from build123d import *

# Parameters (mm, degrees)
SKETCH_1_W      = 215
SKETCH_1_H      = 43.5
EXTRUDE_1_DEPTH = 26
SKETCH_2_W      = 12
SKETCH_2_H      = 20
SKETCH_2_R      = 3.5
EXTRUDE_2_DEPTH = 5
SKETCH_3_R      = 4.2
EXTRUDE_3_DEPTH = 25


with BuildPart() as part:
    # ｽｹｯﾁ1 → ﾎﾞｽ - 押し出し1 (new body)
    with BuildSketch(Plane(origin=(0, 0, 0), x_dir=(1, 0, 0), z_dir=(0, 1, 0))):
        Rectangle(SKETCH_1_W, SKETCH_1_H)
    extrude(amount=EXTRUDE_1_DEPTH)

    # ｽｹｯﾁ2 → ﾎﾞｽ - 押し出し2 (add)
    # profile 1 of 2: a face of its own
    with BuildSketch(Plane.XZ):
        with Locations((-113.5, 0)):
            Rectangle(SKETCH_2_W, SKETCH_2_H)
        with Locations(Location((-113.5, 0, 0), (0, 0, 270))):
            Circle(SKETCH_2_R, mode=Mode.SUBTRACT)
    # profile 2 of 2: a face of its own
    with BuildSketch(Plane.XZ):
        with Locations((113.5, 0)):
            Rectangle(SKETCH_2_W, SKETCH_2_H)
        with Locations(Location((113.5, 0, 0), (0, 0, 90))):
            Circle(SKETCH_2_R, mode=Mode.SUBTRACT)
    extrude(amount=-EXTRUDE_2_DEPTH)

    # ｽｹｯﾁ3 → ﾎﾞｽ - 押し出し3 (add)
    with BuildSketch(Plane.ZY.offset(107.5)):
        with Locations(Location((-7.75, 14, 0), (0, 0, 180))):
            Circle(SKETCH_3_R)
    extrude(amount=EXTRUDE_3_DEPTH)


solid = part.part
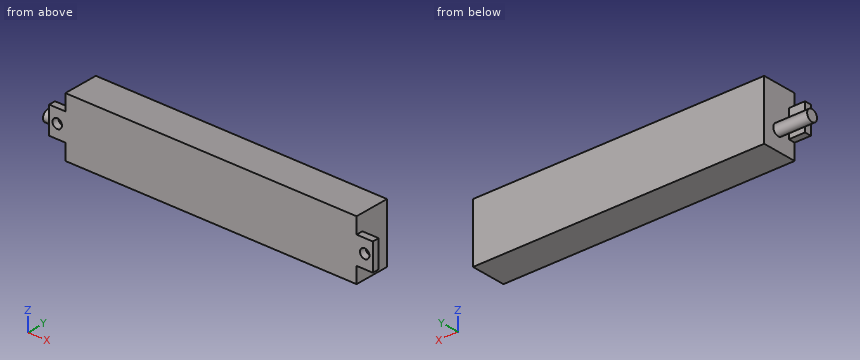
Read the model definition and answer for the solid it produces. Units are mm, in the model's axes. Coordinates: 2 decimals unless noted, no trailing zeros. Order: outer loops, then holes, each group sorted by start corner. A loop starts at its lowest first (then second) coordinate and runs counter-clockwise, first axis right, second up. Notation, with made-up numbers: (-8, 41) - (26, 41) arc R22 cw to (26, 55) - close; hole circle Ø1 at (-4, -21). An arc over 180 degrees is marked (long way). Use one line per item in the form item = value.
(1) Straight lines are drawn through the part: L1, parallel to X at y = 3.4, z = 0; L2, parallel to Z at x = 113.5, y = 3.4; L3, parallel to X at y = 15, z = -16. For each, find the intervals that lie inside material, in ascending order.
Computed values:
L1 = -119.5 to -117, -110 to 110, 117 to 119.5
L2 = -10 to -3.5, 3.5 to 10
L3 = -107.5 to 107.5
(2) Section C-C, the plane y = 14 is taken. Give the vertices of the cut face in (x, z), then the cut area to 3 significant figures.
Computed values:
outline = (-132.5, -11.95) - (-107.5, -11.95) - (-107.5, -21.75) - (107.5, -21.75) - (107.5, 21.75) - (-107.5, 21.75) - (-107.5, -3.55) - (-132.5, -3.55) - close
area = 9,560 mm²
(3) Section B-B, the plane x = 113.5 is taken. Give the vertices of the cut face in (y, z), then the cut area to 3 significant figures.
Computed values:
outline = (0, -10) - (5, -10) - (5, -3.5) - (0, -3.5) - close; (0, 3.5) - (5, 3.5) - (5, 10) - (0, 10) - close
area = 65.0 mm²
(4) Given pin 1 Ø6 at (y, z) = (5.5, -17.5) entering from +X; pin 2 Ø3.5 at (x, z) = (-112.5, 1.5) entering from +Y; pin 3 Ø2.5 at (x, y) = (114.5, 1.5) entering from -Z; pin 4 Ø9 at (x, z) = (-113.5, 0) entering from -Y, each flat-ended and moving along its own axis, determine where each tip first touches the part or whether it passes through.
Computed values:
pin_1 = 107.5
pin_2 = 5
pin_3 = -10
pin_4 = 0
(5) Section D-D, the plane z = -7.75 is taken. Give the vertices of the cut face in (x, y).
Computed values:
outline = (-132.5, 9.8) - (-107.5, 9.8) - (-107.5, 5) - (-119.5, 5) - (-119.5, 0) - (119.5, 0) - (119.5, 5) - (107.5, 5) - (107.5, 26) - (-107.5, 26) - (-107.5, 18.2) - (-132.5, 18.2) - close
(6) Section A-A, the plane x = -113.5 is taken. Give the vertices of the cut face in (y, z), then the cut area to 3 significant figures.
Computed values:
outline = (0, -10) - (5, -10) - (5, -3.5) - (0, -3.5) - close; (0, 3.5) - (5, 3.5) - (5, 10) - (0, 10) - close; circle Ø8.4 at (14, -7.75)
area = 120 mm²
